Study the drawing (mm; zero at the part's minimum x, y, z) and answer. Round coordinates to 2 decimals unless told otherwise and drop trailing zeros. Loops run counter-clockwise (first coordinate to the right, second up) from the corner with the lowest first, then second, coordinate; pieces in that order, holes last. Notation, with made-up numbers: M 79,32.25 L 135,32.25 A33 ccw 135,66.25 Z; hole C 85.25,82 d11. An arc over 180 degrees is marked long. Write each question's results on one line, items separated by ' | '.
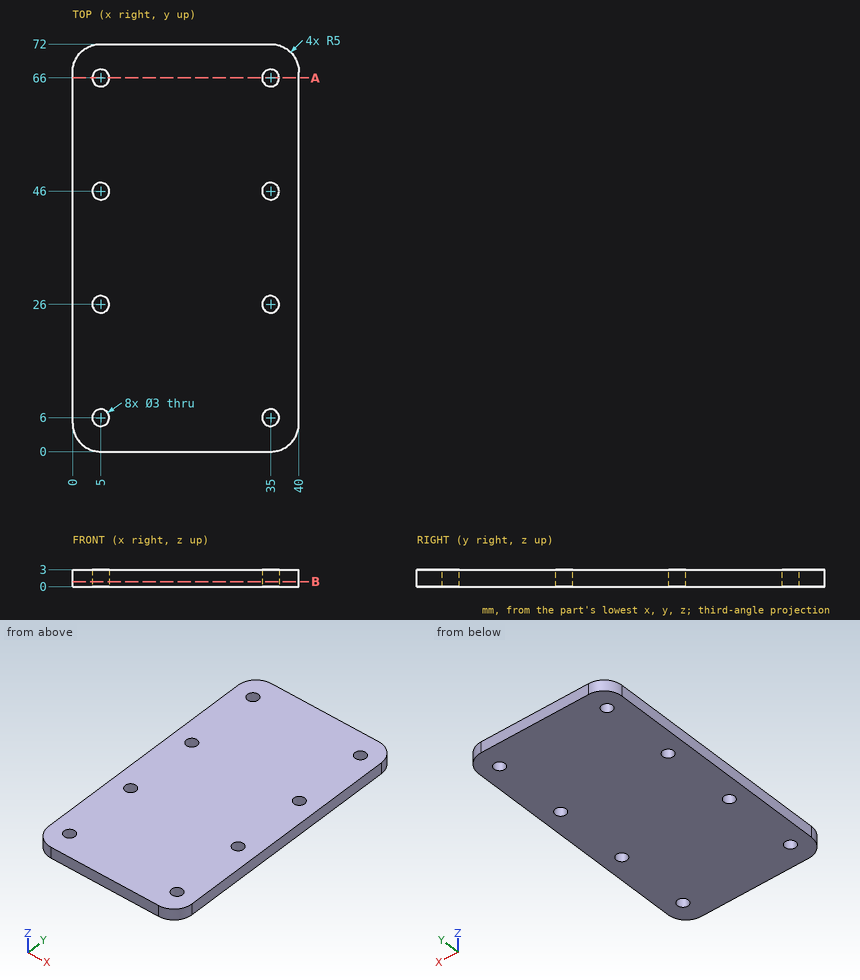
Item 1: Straight lines are drawn through the part: line 1 (Y direction, x = 5, z = 1.95); line 2 (X direction, y = 66, z = 2.1); line 3 (X direction, y = 45.5, z = 1.7). For each, find the intervals that lie inside material, in ascending order.
Outcome:
line 1: y = 0 to 4.5, 7.5 to 24.5, 27.5 to 44.5, 47.5 to 64.5, 67.5 to 72 | line 2: x = 0 to 3.5, 6.5 to 33.5, 36.5 to 40 | line 3: x = 0 to 3.59, 6.41 to 33.59, 36.41 to 40
Item 2: The part is cut by section A-A (y = 66). Determine the outline of the cut face in (x, z).
Outcome:
outline: M 0,0 L 3.5,0 L 3.5,3 L 0,3 Z; M 6.5,0 L 33.5,0 L 33.5,3 L 6.5,3 Z; M 36.5,0 L 40,0 L 40,3 L 36.5,3 Z
Item 3: The part is cut by section B-B (z = 0.85). State how many separate pieces and enclosed holes the cut face has, plus the area to 3 significant figures.
Outcome:
separate pieces: 1 | enclosed holes: 8 | area: 2,800 mm2
Item 4: A flat-ended cylindrical pin translates along its axis: pin 1 (5 mm diameter, centred on x = 5, y = 6, fed in from +Z). Find the tip coordinate at first contact, or state that the pin passes through.
Outcome:
pin 1: stops at z = 3
